The model under review builds one solid part; all positions refer to its coordinate system, in mm. A direction names the side the tool comes from. Coordinates: 2 decimals unless noted, no trailing zeros. Order: outer loops, then holes, each group sorted by start corner. A loop starts at its lowest first (then second) coordinate and runs counter-clockwise, first axis right, second up. Notation, with made-up numbers: M 69.5,49 L 84.5,49 A6 ccw 84.5,53 Z; hole C 8.25,-16.5 d9. An arc over 180 degrees is marked long. Write each question's results on one line, items separated by ' | '.
from build123d import *

# Parameters (mm, degrees)
SKETCH2_W           = 37.5
SKETCH2_H           = 37.5
SKETCH2_R           = 15
BOSS_EXTRUDE1_DEPTH = 23
SKETCH3_R           = 15
BOSS_EXTRUDE2_DEPTH = 3
FILLET2_R           = 3
FILLET3_R           = 2


with BuildPart() as part:
    # Sketch1 → Revolve1 (revolve)
    with BuildSketch(Plane.XY, mode=Mode.PRIVATE) as revolve1_sk:
        with BuildLine():
            Line((0, 10), (21.139278074, 10))
            ThreePointArc((21.139278074, 10), (42.204515534, 18.013203992), (55.75, 0))
            Line((55.75, 0), (0, 0))
            Line((0, 0), (0, 10))
        make_face()
    revolve(revolve1_sk.sketch.rotate(Axis((55.75, 0, 0), (-1, 0, 0)), 180), axis=Axis((55.75, 0, 0), (-1, 0, 0)))



with BuildPart() as body_2:
    # Sketch2 → Boss-Extrude1 (new body)
    with BuildSketch(Plane.ZY):
        Rectangle(SKETCH2_W, SKETCH2_H)
        Circle(SKETCH2_R, mode=Mode.SUBTRACT)
    extrude(amount=BOSS_EXTRUDE1_DEPTH)


with BuildPart() as part_1:
    add(part.part)

    add(body_2.part)  # Boss-Extrude2 merges body 2
    # Sketch3 → Boss-Extrude2 (add)
    with BuildSketch(Plane.ZY):
        Circle(SKETCH3_R)
    extrude(amount=BOSS_EXTRUDE2_DEPTH)

    # Fillet2
    fillet2_edges = [part_1.edges().sort_by_distance(p)[0] for p in [
        (0, 10, 0),
        (0, 0, 18.75),
        (-11.5, -18.75, 18.75),
        (0, 18.75, 0),
        (-11.5, 18.75, 18.75),
        (0, 0, -18.75),
        (-11.5, 18.75, -18.75),
        (0, -18.75, 0),
        (-11.5, -18.75, -18.75),
        (21.139278074, 10, 0),
    ]]
    fillet(fillet2_edges, radius=FILLET2_R)

    # Fillet3
    fillet3_edges = [part_1.edges().sort_by_distance(p)[0] for p in [
        (-23, 0, -15),
    ]]
    fillet(fillet3_edges, radius=FILLET3_R)


solid = part_1.part
1) Take a section at C-C on x = 30. State the section outline as (y, z) points.
Solutions:
outline: C 0,0 d34.79
2) To check wall thickness, follow line 1 along Y through (x, z) = (-10, 0); line 2 along X through (y, z) = (16, -13); line 3 along X through (y, z) = (11, 11.5). State the ranges of each line that lie inside material, in increasing order.
Solutions:
line 1: -18.75 to -15, 15 to 18.75 | line 2: -23 to -0.01 | line 3: -22.68 to 0, 27.08 to 46.92
3) Take a section at A-A on x = -5.5. State the section outline as (y, z) points.
Solutions:
outline: M -18.75,-15.75 A3 ccw -15.75,-18.75 L 15.75,-18.75 A3 ccw 18.75,-15.75 L 18.75,15.75 A3 ccw 15.75,18.75 L -15.75,18.75 A3 ccw -18.75,15.75 Z; hole C 0,0 d30
4) The part is to be moulded in two halves that separate along Y. For faces 1 (the flat face through (-3, 0, 0)), 2 (the flat face through (-23, -4, -17)), 3 (the cylindrical face through (-13.14, -17.89, 17.85)), say which applies: pulls with the +Y half, pulls with the -Y half, needs draft (parallel to the pull), parting line crosses it, or undercut.
Solutions:
face 1: undercut | face 2: needs draft | face 3: pulls with the -Y half
5) For pin 1 (8 mm diameter, centred on x = 11.5, y = -7, fed in from -Z); pin 2 (1 mm diameter, centred on x = 22.5, y = 5, fed in from +Z); pin 3 (1.5 mm diameter, centred on y = 11.5, z = -4, fed in from +X), all flat-tipped, find the tip position at first contact; note any pin that passes through.
Solutions:
pin 1: z = -9.54 | pin 2: z = 11.46 | pin 3: x = 51.87
6) For faces 4 (the flat face through (0, 0, 14)), 5 (the cylindrical face through (-0.86, -17.85, 0.22)), 6 (the cylindrical face through (-11.874, 0.66, -14.985)), 7 (the cylindrical face through (-0.86, 0.22, 17.85)), 8 (the cylindrical face through (-0.86, 17.85, 0.22)), list the 3-axis set-ups (+Z, -Z, +X, -X, +Y, -Y) from which the entire face can be reached by the end or side of a thin tool; tool diameter is ignored.
Solutions:
face 4: none | face 5: +Z, -Z, -Y | face 6: -X | face 7: +Z, +Y, -Y | face 8: +Z, -Z, +Y
7) Take a section at B-B on x = 6.5. State the section outline as (y, z) points, plus the area to 3 significant figures.
Solutions:
outline: C 0,0 d20 | area: 314 mm2
